Geometry check sheet. Reference: drawing and pictorial views, mm from the part's lowest x, y, z. A direction names the side the tool comes from. Coordinates: 2 decimals unless noted, no trailing zeros. Loops run counter-clockwise (first coordinate to the right, second up) from the corner with the lowest first, then second, coordinate; pieces in that order, holes last. Notation, with made-up numbers: (-26, -20) - (-12, -20) arc R18 ccw to (-12, 10) - close; hole circle Ø11 at (-35.75, 44). An arc over 180 degrees is marked (long way). Use a Markdown table: item, result. Add a question column.
1) Sectioned sample at D-D, the plane x = 243. Enter the section's corners in (y, z).
2) Sectioned sample at A-A, the plane y = 36.5. Enter the section's corners in (x, z) (1 decimal).
3) Go/stop test with flat-tipped pins: P1, Ø18, axis at y = 40, z = 9.5, coming from the -X side; P2, Ø19, axis at x = 79.5, z = 35, coming from the +Y side. Record where each tip stops, or that it passes through.
4) Thickness scan on line 1 (Y direction, x = 117, z = 10.5); line 2 (X direction, y = 24, z = 66) (1 decimal); line 3 (X direction, y = 9, z = 32). Record the ranges inside material, lowest first.
5) Sectioned sample at C-C, the plane z = 54.5. Enter the section's corners in (x, y) (1 decimal).
6) Tool access check on the marked faces 5 and 6. Record the directions out of +Z, -Z, +X, -X, +Y, -Y that give a thin tool (end or side, any length) a straight path to the whole face; none if there is none.
7) Draft check along X on the marked faces 1, 2, 3 and 4. Enter one of: pulls with the +X half, pulls with the -X half, needs draft (parallel to the pull), parting line crosses it, or undercut.
8) Sectioned sample at B-B, the plane x = 100.5. Enter the section's corners in (y, z).
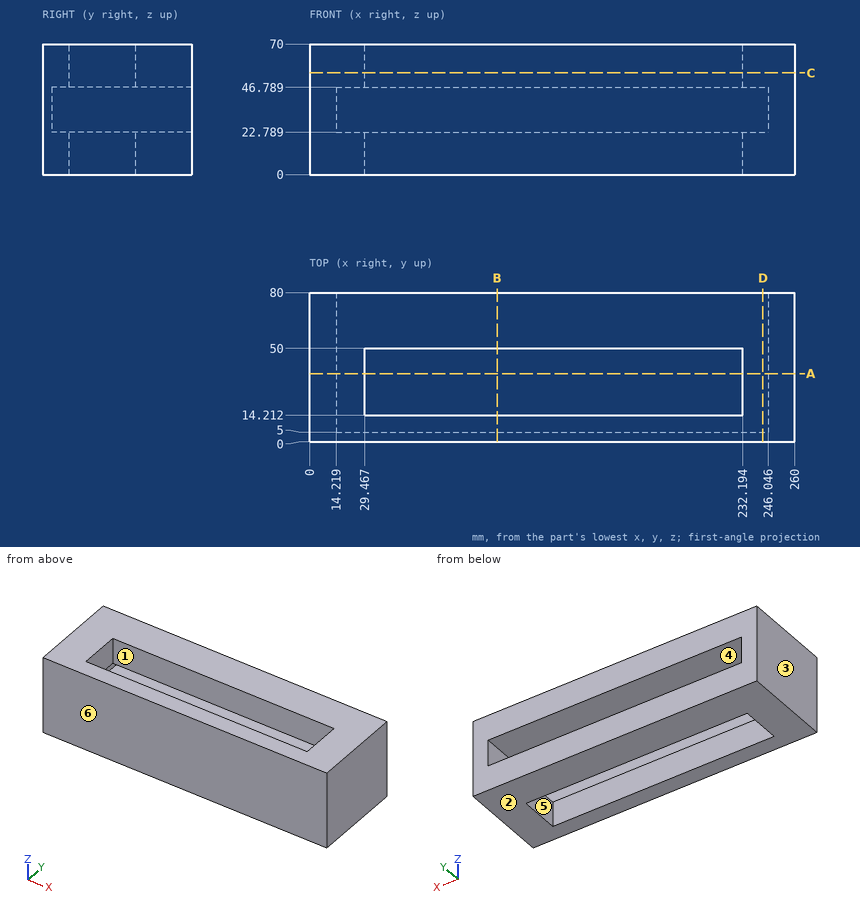
Solved:
| question | item | result |
|---|---|---|
| 1 | outline | (0, 0) - (80, 0) - (80, 22.79) - (5, 22.79) - (5, 46.79) - (80, 46.79) - (80, 70) - (0, 70) - close |
| 2 | outline | (0, 0) - (29.5, 0) - (29.5, 22.8) - (14.2, 22.8) - (14.2, 46.8) - (29.5, 46.8) - (29.5, 70) - (0, 70) - close; (232.2, 0) - (260, 0) - (260, 70) - (232.2, 70) - (232.2, 46.8) - (246, 46.8) - (246, 22.8) - (232.2, 22.8) - close |
| 3 | P1 | stops at x = 0 |
| 3 | P2 | stops at y = 5 |
| 4 | line 1 | y = 0 to 14.21, 50 to 80 |
| 4 | line 2 | x = 0 to 29.5, 232.2 to 260 |
| 4 | line 3 | x = 0 to 14.22, 246.05 to 260 |
| 5 | outline | (0, 0) - (260, 0) - (260, 80) - (0, 80) - close; hole (29.5, 14.2) - (232.2, 14.2) - (232.2, 50) - (29.5, 50) - close |
| 6 | face 5 | +Z, -Z |
| 6 | face 6 | +Z, -Z, +X, -X, -Y |
| 7 | face 1 | undercut |
| 7 | face 2 | needs draft |
| 7 | face 3 | pulls with the -X half |
| 7 | face 4 | undercut |
| 8 | outline | (0, 0) - (14.21, 0) - (14.21, 22.79) - (5, 22.79) - (5, 46.79) - (14.21, 46.79) - (14.21, 70) - (0, 70) - close; (50, 0) - (80, 0) - (80, 22.79) - (50, 22.79) - close; (50, 46.79) - (80, 46.79) - (80, 70) - (50, 70) - close |
